```python
from build123d import *

# Parameters (mm, degrees)
BOSS_EXTRUDE1_DEPTH     = 4.2
CUT_EXTRUDE4_DEPTH      = 62.783185415
CUT_EXTRUDE4_DEPTH_BACK = 62.783185415
SKETCH2_R               = 1.6
SKETCH3_W               = 4
SKETCH3_H               = 14
CUT_EXTRUDE5_DEPTH      = 62.783185415
SKETCH6_W               = 31.08
SKETCH6_H               = 48.86
CUT_EXTRUDE6_DEPTH      = 1.6
CUT_EXTRUDE7_DEPTH      = 65.562744675
CUT_EXTRUDE7_DEPTH_BACK = 35
CUT_EXTRUDE8_DEPTH      = 62.695072737
CUT_EXTRUDE8_DEPTH_BACK = 62.695072737
SKETCH9_R               = 3.5


with BuildPart() as part:
    # Sketch1 → Boss-Extrude1 (new body)
    with BuildSketch(Plane(origin=(0, 0, 0), x_dir=(1, 0, 0), z_dir=(0, 1, 0))):
        with BuildLine():
            Line((-3.3, -0.3), (-3.3, 48.56))
            ThreePointArc((-3.3, 48.56), (-2.421320344, 50.681320344), (-0.3, 51.56))
            Line((-0.3, 51.56), (30.78, 51.56))
            ThreePointArc((30.78, 51.56), (32.901320344, 50.681320344), (33.78, 48.56))
            Line((33.78, 48.56), (33.78, -0.3))
            ThreePointArc((33.78, -0.3), (32.901320344, -2.421320344), (30.78, -3.3))
            Line((30.78, -3.3), (-0.3, -3.3))
            ThreePointArc((-0.3, -3.3), (-2.421320344, -2.421320344), (-3.3, -0.3))
        make_face()
    extrude(amount=BOSS_EXTRUDE1_DEPTH)

    # Sketch2 → Cut-Extrude4 (cut, two sides: drawn at the far end of the back side and taken through both)
    with BuildSketch(Plane(origin=(0, 0, 0), x_dir=(1, 0, 0), z_dir=(0, 1, 0)).offset(-CUT_EXTRUDE4_DEPTH_BACK)):
        with Locations(Location((3.81, 43.18, 0), (0, 0, 270))):
            Circle(SKETCH2_R)
        with Locations(Location((26.67, 43.18, 0), (0, 0, 270))):
            Circle(SKETCH2_R)
        with Locations(Location((15.24, 3.81, 0), (0, 0, 270))):
            Circle(SKETCH2_R)
    extrude(amount=CUT_EXTRUDE4_DEPTH + CUT_EXTRUDE4_DEPTH_BACK, mode=Mode.SUBTRACT)

    # Sketch3 → Cut-Extrude5 (cut, through all)
    with BuildSketch(Plane(origin=(0, 0, 0), x_dir=(1, 0, 0), z_dir=(0, 1, 0))):
        with Locations((2.54, 16.51)):
            Rectangle(SKETCH3_W, SKETCH3_H)
        with Locations((27.94, 16.51)):
            Rectangle(SKETCH3_W, SKETCH3_H)
    extrude(amount=CUT_EXTRUDE5_DEPTH, mode=Mode.SUBTRACT)

    # Sketch6 → Cut-Extrude6 (cut)
    with BuildSketch(Plane(origin=(0, 4.2, 0), x_dir=(1, 0, 0), z_dir=(0, 1, 0))):
        with Locations((15.24, 24.13)):
            Rectangle(SKETCH6_W, SKETCH6_H)
    extrude(amount=-CUT_EXTRUDE6_DEPTH, mode=Mode.SUBTRACT)

    # Sketch8 → Cut-Extrude7 (cut, two sides: drawn at the far end of the back side and taken through both)
    with BuildSketch(Plane.XY.offset(3.3).offset(-CUT_EXTRUDE7_DEPTH_BACK)):
        with BuildLine():
            ThreePointArc((1.74, 0), (1.542515791, 0.67088902), (1.832893219, 1.307106781))
            Line((1.832893219, 1.307106781), (0.54, 0.014213562))
            Line((0.54, 0.014213562), (0.54, 0))
            Line((0.54, 0), (1.74, 0))
        make_face()
        with BuildLine():
            ThreePointArc((1.832893219, 1.307106781), (2.54, 1.6), (3.247106781, 1.307106781))
            Line((3.247106781, 1.307106781), (2.54, 2.014213562))
            Line((2.54, 2.014213562), (1.832893219, 1.307106781))
        make_face()
        with BuildLine():
            ThreePointArc((3.54, 0.6), (3.463879533, 0.982683432), (3.247106781, 1.307106781))
            ThreePointArc((3.247106781, 1.307106781), (2.54, 1.6), (1.832893219, 1.307106781))
            ThreePointArc((1.832893219, 1.307106781), (1.542515791, 0.67088902), (1.74, 0))
            Line((1.74, 0), (3.34, 0))
            ThreePointArc((3.34, 0), (3.488683298, 0.283772234), (3.54, 0.6))
        make_face()
        with BuildLine():
            ThreePointArc((1.74, 0), (2.54, -0.4), (3.34, 0))
            Line((3.34, 0), (1.74, 0))
        make_face()
        with BuildLine():
            Line((4.54, 0), (4.54, 0.014213562))
            Line((4.54, 0.014213562), (3.247106781, 1.307106781))
            ThreePointArc((3.247106781, 1.307106781), (3.463879533, 0.982683432), (3.54, 0.6))
            ThreePointArc((3.54, 0.6), (3.488683298, 0.283772234), (3.34, 0))
            Line((3.34, 0), (4.54, 0))
        make_face()
        with BuildLine():
            Line((29.94, 0.014213562), (28.647106781, 1.307106781))
            ThreePointArc((28.647106781, 1.307106781), (28.863879533, 0.982683432), (28.94, 0.6))
            ThreePointArc((28.94, 0.6), (28.888683298, 0.283772234), (28.74, 0))
            Line((28.74, 0), (29.94, 0))
            Line((29.94, 0), (29.94, 0.014213562))
        make_face()
        with BuildLine():
            Line((28.647106781, 1.307106781), (27.94, 2.014213562))
            Line((27.94, 2.014213562), (27.23289323, 1.307106792))
            ThreePointArc((27.23289323, 1.307106792), (27.940000008, 1.6), (28.647106781, 1.307106781))
        make_face()
        with BuildLine():
            ThreePointArc((28.94, 0.6), (28.863879533, 0.982683432), (28.647106781, 1.307106781))
            ThreePointArc((28.647106781, 1.307106781), (27.940000008, 1.6), (27.23289323, 1.307106792))
            ThreePointArc((27.23289323, 1.307106792), (26.942515792, 0.670889028), (27.14, 0))
            Line((27.14, 0), (28.74, 0))
            ThreePointArc((28.74, 0), (28.888683298, 0.283772234), (28.94, 0.6))
        make_face()
        with BuildLine():
            Line((28.74, 0), (27.14, 0))
            ThreePointArc((27.14, 0), (27.94, -0.4), (28.74, 0))
        make_face()
        with BuildLine():
            ThreePointArc((27.14, 0), (26.942515792, 0.670889028), (27.23289323, 1.307106792))
            Line((27.23289323, 1.307106792), (25.94, 0.014213562))
            Line((25.94, 0.014213562), (25.94, 0))
            Line((25.94, 0), (27.14, 0))
        make_face()
    extrude(amount=CUT_EXTRUDE7_DEPTH + CUT_EXTRUDE7_DEPTH_BACK, mode=Mode.SUBTRACT)

    # Sketch9 → Cut-Extrude8 (cut, two sides: drawn at the far end of the back side and taken through both)
    with BuildSketch(Plane(origin=(0, 2.6, 0), x_dir=(1, 0, 0), z_dir=(0, 1, 0)).offset(-CUT_EXTRUDE8_DEPTH_BACK)):
        with Locations(Location((15.24, 25.4, 0), (0, 0, 270))):
            Circle(SKETCH9_R)
        with BuildLine():
            Line((8.24, 44.68), (22.24, 44.68))
            ThreePointArc((22.24, 44.68), (23.74, 43.18), (22.24, 41.68))
            Line((22.24, 41.68), (8.24, 41.68))
            ThreePointArc((8.24, 41.68), (6.74, 43.18), (8.24, 44.68))
        make_face()
    extrude(amount=CUT_EXTRUDE8_DEPTH + CUT_EXTRUDE8_DEPTH_BACK, mode=Mode.SUBTRACT)


solid = part.part
```
Could you check a few things on this model? Use its own coordinates, in mm. A direction names the side the tool comes from. Round coordinates to 2 decimals unless told otherwise and drop trailing zeros. Write each loop counter-clockwise with the first axis right and the second up, starting at its lowest first coordinate (ties: lowest second). Pieces come first, ordered by that corner, then holes. Notation, with made-up numbers: M 8.5,75 L 57.5,75 A22 ccw 57.5,99 Z; hole C 28.5,35 d3. An arc over 180 degrees is marked long. Answer in a Markdown table with one row per item. Add a question column.
Q1. Will these pins go through, and if not, where does the flat tip stop? pin 1 Ø1 at (x, y) = (3, 0.5) entering from +Z; pin 2 Ø1.5 at (x, z) = (3.5, -43.5) entering from -Y; pin 3 Ø11 at (x, z) = (15.24, -25.4) entering from +Y.
Q2. If I drill on line 1 (X direction, y = 1.55, z = -13); line 2 (Z direction, x = 3.81, y = 2); line 3 (X direction, y = 1.3, z = -31), over which ranges is the centre line in solid material (lowest first)? Write a range as from..to.
Q3. On a 3-axis mill with a long thin cutter (end or side, diameter ignored), from which of +Z, -Z, +X, -X, +Y, -Y can I reach the whole of each face in a straight line? I mean faces 4 (the cylindrical face through (32.92, 2.07, 2.4)), 5 (the flat face through (26.954, 1.028, -27.662)), 6 (the flat face through (30.78, 3, -24)), 7 (the flat face through (27, 2, -9.51)). Say none if no direction works.
Q4. Imagine slicing it at C-C (x = 15.24). Please give me the cut outline in (y, z).
Q5. Imagine slicing it at D-D (z = -16). Please give me the cut outline in (x, y), then the cut area to 3 significant figures.
Q6. Imagine slicing it at B-B (y = 3.5). Please give me the cut outline in (x, z), then the cut area to 3 significant figures.
Q7. If we mould it in two halves opening along Z, with no side actions, what happens to faces 1 (the flat face through (15, 2, 3.3)), 2 (the flat face through (15, 1, -44.68)), 3 (the flat face through (28.954, 1, -3.195))? For each: +Z half, -Z half, draft (parallel to the pull), parting line (faces both ways), or undercut.
Values:
| question | item | result |
|---|---|---|
| 1 | pin 1 | z = -31.7 |
| 1 | pin 2 | through |
| 1 | pin 3 | y = 2.6 |
| 2 | line 1 | -3.3..0.54, 4.54..25.94, 29.94..33.78 |
| 2 | line 2 | -51.56..-44.78, -41.58..-23.51, -9.51..3.3 |
| 2 | line 3 | -3.3..1.83, 3.25..27.23, 28.65..33.78 |
| 3 | face 4 | +Z, +X, +Y, -Y |
| 3 | face 5 | +Z, -Y |
| 3 | face 6 | +Y |
| 3 | face 7 | +Y, -Y |
| 4 | outline | M 0,-51.56 L 4.2,-51.56 L 4.2,-48.56 L 2.6,-48.56 L 2.6,-44.68 L 0,-44.68 Z; M 0,-41.68 L 2.6,-41.68 L 2.6,-28.9 L 0,-28.9 Z; M 0,-21.9 L 2.6,-21.9 L 2.6,-5.41 L 0,-5.41 Z; M 0,-2.21 L 2.6,-2.21 L 2.6,0.3 L 4.2,0.3 L 4.2,3.3 L 0,3.3 Z |
| 5 | outline | M -3.3,0 L 0.54,0 L 0.54,2.6 L -0.3,2.6 L -0.3,4.2 L -3.3,4.2 Z; M 4.54,0 L 25.94,0 L 25.94,2.6 L 4.54,2.6 Z; M 29.94,0 L 33.78,0 L 33.78,4.2 L 30.78,4.2 L 30.78,2.6 L 29.94,2.6 Z |
| 5 | area | 85.2 mm^2 |
| 6 | outline | M -3.3,-48.56 A3 ccw -0.3,-51.56 L 30.78,-51.56 A3 ccw 33.78,-48.56 L 33.78,0.3 A3 ccw 30.78,3.3 L -0.3,3.3 A3 ccw -3.3,0.3 Z; hole M -0.3,-48.56 L 30.78,-48.56 L 30.78,0.3 L -0.3,0.3 Z |
| 6 | area | 508 mm^2 |
| 7 | face 1 | +Z half |
| 7 | face 2 | undercut |
| 7 | face 3 | draft |
